Source: CAD feature listing. Evaluate the final solid. Frame: model axes, mm. A direction names the side the tool comes from. Give positions to 0.01 mm unless a question says otherwise; leave off trailing zeros. Write each loop counter-clockwise with the first axis right and the second up, starting at its lowest first coordinate (ties: lowest second). Pieces come first, ordered by that corner, then holes.
```python
from build123d import *

# Parameters (mm, degrees)
SKETCH1_W           = 37.4
SKETCH1_H           = 22.5
SKETCH1_R           = 1
SKETCH1_W_2         = 22.4
SKETCH1_H_2         = 12.5
BOSS_EXTRUDE1_DEPTH = 7.46
SKETCH2_W           = 31.8
SKETCH2_H           = 12.5
CUT_EXTRUDE1_DEPTH  = 2
SKETCH3_R           = 2.5
CUT_EXTRUDE2_DEPTH  = 25.380404016
SKETCH4_R           = 3.05
CUT_EXTRUDE3_DEPTH  = 0.7
CUT_EXTRUDE4_START  = -0.7
SKETCH5_R           = 3.05
CUT_EXTRUDE4_DEPTH  = 0.7


with BuildPart() as part:
    # Sketch1 → Boss-Extrude1 (new body)
    with BuildSketch(Plane(origin=(0, 0, 0), x_dir=(1, 0, 0), z_dir=(0, 1, 0))):
        with Locations((0, 2.5)):
            Rectangle(SKETCH1_W, SKETCH1_H)
        with Locations(Location((13.85, 0, 0), (0, 0, 270))):
            Circle(SKETCH1_R, mode=Mode.SUBTRACT)
        with Locations(Location((-13.85, 0, 0), (0, 0, 270))):
            Circle(SKETCH1_R, mode=Mode.SUBTRACT)
        Rectangle(SKETCH1_W_2, SKETCH1_H_2, mode=Mode.SUBTRACT)
    extrude(amount=-BOSS_EXTRUDE1_DEPTH)

    # Sketch2 → Cut-Extrude1 (cut)
    with BuildSketch(Plane(origin=(0, 0, 0), x_dir=(1, 0, 0), z_dir=(0, 1, 0))):
        Rectangle(SKETCH2_W, SKETCH2_H)
    extrude(amount=-CUT_EXTRUDE1_DEPTH, mode=Mode.SUBTRACT)

    # Sketch3 → Cut-Extrude2 (cut, through all)
    with BuildSketch(Plane(origin=(0, 0, 0), x_dir=(1, 0, 0), z_dir=(0, 1, 0))):
        with Locations(Location((8, 10, 0), (0, 0, 270))):
            Circle(SKETCH3_R)
        with Locations(Location((-8, 10, 0), (0, 0, 270))):
            Circle(SKETCH3_R)
    extrude(amount=-CUT_EXTRUDE2_DEPTH, mode=Mode.SUBTRACT)

    # Sketch4 → Cut-Extrude3 (cut)
    with BuildSketch(Plane(origin=(0, 0, 0), x_dir=(1, 0, 0), z_dir=(0, 1, 0))):
        with Locations(Location((-8, 10, 0), (0, 0, 270))):
            Circle(SKETCH4_R)
        with Locations(Location((8, 10, 0), (0, 0, 270))):
            Circle(SKETCH4_R)
    extrude(amount=-CUT_EXTRUDE3_DEPTH, mode=Mode.SUBTRACT)

    # Sketch5 → Cut-Extrude4 (cut)
    with BuildSketch(Plane(origin=(0, -7.46, 0), x_dir=(-1, 0, 0), z_dir=(0, -1, 0)).offset(CUT_EXTRUDE4_START)):
        with Locations(Location((-8, 10, 0), (0, 0, 270))):
            Circle(SKETCH5_R)
        with Locations(Location((8, 10, 0), (0, 0, 270))):
            Circle(SKETCH5_R)
    extrude(amount=CUT_EXTRUDE4_DEPTH, mode=Mode.SUBTRACT)


solid = part.part
```
1. Section query A-A (z = -10). Return loops of the section in (x, y), plus the area to 3 significant figures.
2. Line query: probe 1 along X at (y, z) = (-7.2, -10); probe 2 along X at (y, z) = (-5.35, 0); probe 3 along Z at (x, y) = (8, -7.25). Output: solid intervals per line, ascending.
3. Section query C-C (x = -13.85). Return loops of the section in (y, z).
4. Pin query (flat end, axial travel): P1, Ø4, axis at x = 12.5, z = 1, coming from the +Y side; P2, Ø3, axis at x = 6.5, z = -11, coming from the -Y side; P3, Ø5.5, axis at x = 8, z = -10, coming from the +Y side. Return the tip coordinate at first contact, or that it passes through.
5. Access query for faces 1 (the flat face through (11.2, -5, 0)), 2 (the flat face through (0, -7.46, -8)), 3 (the cylindrical face through (-8.134, -7.105, -13.047)), 4 (the flat face through (-12.5, -2, -0.1)), 5 (the flat face through (0, -4, 8.75)). Directions: +Z, -Z, +X, -X, +Y, -Y. A direction counts if a zero-diameter tool reaches every point of the face in a straight line with its end or side. Return the directions, or none.
6. Section query B-B (x = 8). Return loops of the section in (y, z), plus the area to 3 significant figures.
7. Pull-direction query (X, two-part tool) for faces 6 (the flat face through (12, -2, 0)), 7 (the flat face through (0, 0, -8)); classes: pulls with the +X half, pulls with the -X half, needs draft (parallel to the pull), parting line crosses it, or undercut.
8. Section query D-D (z = 0). Return loops of the section in (x, y).
The answers:
1. outline: (-18.7, -7.46) - (-11.05, -7.46) - (-11.05, -6.76) - (-10.5, -6.76) - (-10.5, -0.7) - (-11.05, -0.7) - (-11.05, 0) - (-18.7, 0) - close; (-5.5, -6.76) - (-4.95, -6.76) - (-4.95, -7.46) - (4.95, -7.46) - (4.95, -6.76) - (5.5, -6.76) - (5.5, -0.7) - (4.95, -0.7) - (4.95, 0) - (-4.95, 0) - (-4.95, -0.7) - (-5.5, -0.7) - close; (10.5, -6.76) - (11.05, -6.76) - (11.05, -7.46) - (18.7, -7.46) - (18.7, 0) - (11.05, 0) - (11.05, -0.7) - (10.5, -0.7) - close
1. area: 201 mm2
2. probe 1: x = -18.7 to -11.05, -4.95 to 4.95, 11.05 to 18.7
2. probe 2: x = -18.7 to -14.85, -12.85 to -11.2, 11.2 to 12.85, 14.85 to 18.7
2. probe 3: z = -13.75 to -13.05, -6.95 to -6.25, 6.25 to 8.75
3. outline: (-7.46, -13.75) - (0, -13.75) - (0, -6.25) - (-2, -6.25) - (-2, -1) - (-7.46, -1) - close; (-7.46, 1) - (-2, 1) - (-2, 6.25) - (0, 6.25) - (0, 8.75) - (-7.46, 8.75) - close
4. P1: stops at y = -2
4. P2: stops at y = -7.46
4. P3: stops at y = -0.7
5. face 1: +Y, -Y
5. face 2: +Z, -Z, +X, -X, -Y
5. face 3: -Y
5. face 4: +Y
5. face 5: +Z, +X, -X, +Y, -Y
6. outline: (-7.46, -13.75) - (0, -13.75) - (0, -13.05) - (-0.7, -13.05) - (-0.7, -12.5) - (-6.76, -12.5) - (-6.76, -13.05) - (-7.46, -13.05) - close; (-7.46, -6.95) - (-6.76, -6.95) - (-6.76, -7.5) - (-0.7, -7.5) - (-0.7, -6.95) - (0, -6.95) - (0, -6.25) - (-7.46, -6.25) - close; (-7.46, 6.25) - (0, 6.25) - (0, 8.75) - (-7.46, 8.75) - close
6. area: 35.8 mm2
7. face 6: undercut
7. face 7: needs draft
8. outline: (-18.7, -7.46) - (-14.85, -7.46) - (-14.85, -2) - (-15.9, -2) - (-15.9, 0) - (-18.7, 0) - close; (-12.85, -7.46) - (-11.2, -7.46) - (-11.2, -2) - (-12.85, -2) - close; (11.2, -7.46) - (12.85, -7.46) - (12.85, -2) - (11.2, -2) - close; (14.85, -7.46) - (18.7, -7.46) - (18.7, 0) - (15.9, 0) - (15.9, -2) - (14.85, -2) - close
